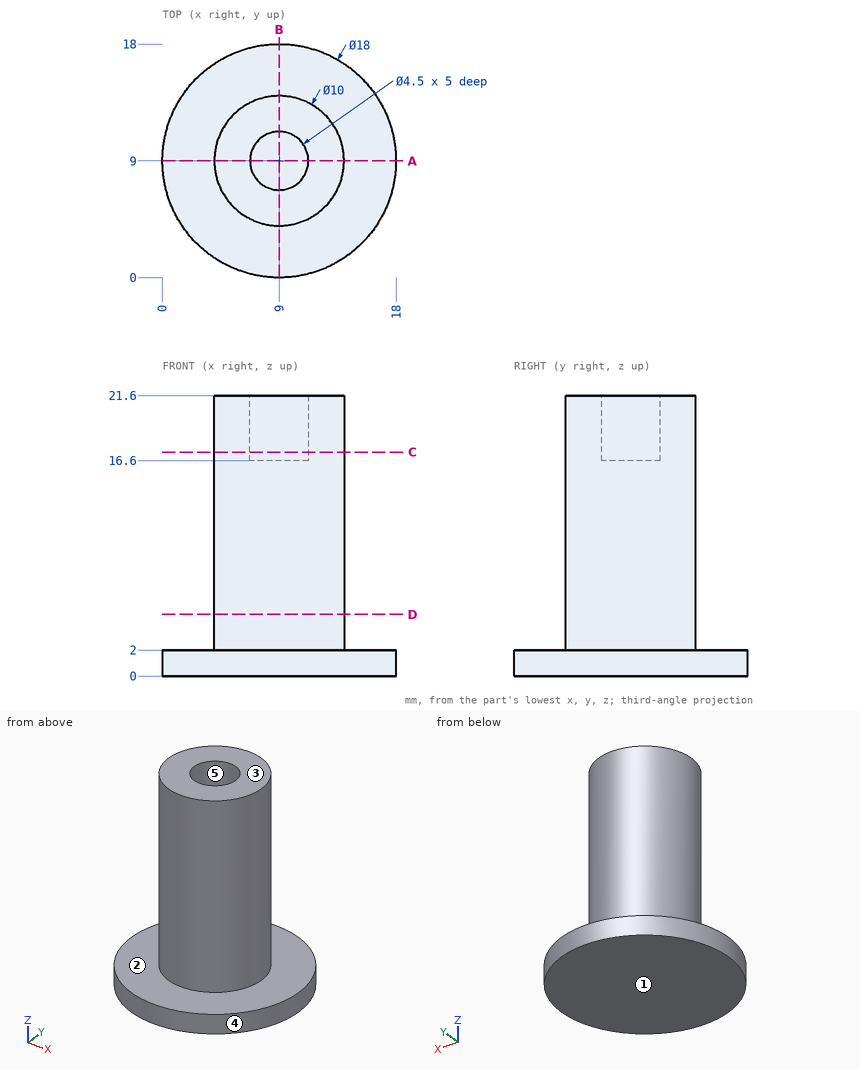
Job drawing, mm, ordinate dimensions from the low corner. One solid piece. A direction names the side the tool comes from. Round coordinates to 2 decimals unless told otherwise and drop trailing zeros. Order: outer loops, then holes, each group sorted by start corner. A loop starts at its lowest first (then second) coordinate and runs counter-clockwise, first axis right, second up. Notation, with made-up numbers: (-2.75, 42) - (35.25, 42) arc R15 cw to (35.25, 71) - close; hole circle Ø1 at (40, 44.25). An arc over 180 degrees is marked (long way). Use CSV: the item, a comma, the result in double quotes. Start each with the question number.
1) Saw through at C-C (z = 17.25). List the corners of the cut face in (x, y), and give its area (3 significant figures).
2) Wall check: L1, parallel to Y at x = 9, z = 17.8; L2, parallel to Z at x = 3.25, y = 14.75; L3, parallel to Z at x = 10, y = 9.5. Give the ranges that are in metal, low to high. Write a range as [from, to].
3) Two-plate mould, pull along Y, no slides. Class the marked faces 3, 4 and 5: pulls with the +Y half, pulls with the -Y half, needs draft (parallel to the pull), parting line crosses it, or undercut.
4) Saw through at D-D (z = 4.75). List the corners of the cut face in (x, y), and give its area (3 significant figures).
5) Tool access for the marked faces 1 and 2: list every direction of +Z, -Z, +X, -X, +Y, -Y with a clear straight run to the whole face (end or side of a thin tool).
6) Pin check, flat tips, straight feed: pin 1 Ø5 at (x, z) = (2, 19) entering from -Y; pin 2 Ø1.5 at (y, z) = (7, 6.5) entering from +X; pin 3 Ø5 at (x, z) = (5.5, 8.5) entering from +Y. Stop position of each tip, or through.
7) Saw through at A-A (y = 9). List the corners of the cut face in (x, z).
Values follow:
1,outline,"circle Ø10 at (9, 9); hole circle Ø4.5 at (9, 9)"
1,area,"62.6 mm2"
2,L1,"y = [4, 6.75], [11.25, 14]"
2,L2,"z = [0, 2]"
2,L3,"z = [0, 16.6]"
3,face 3,"needs draft"
3,face 4,"parting line crosses it"
3,face 5,"undercut"
4,outline,"circle Ø10 at (9, 9)"
4,area,"78.5 mm2"
5,face 1,"-Z, +X, -X, +Y, -Y"
5,face 2,"+Z"
6,pin 1,"stops at y = 6.82"
6,pin 2,"stops at x = 13.84"
6,pin 3,"stops at y = 13.9"
7,outline,"(0, 0) - (18, 0) - (18, 2) - (14, 2) - (14, 21.6) - (11.25, 21.6) - (11.25, 16.6) - (6.75, 16.6) - (6.75, 21.6) - (4, 21.6) - (4, 2) - (0, 2) - close"
